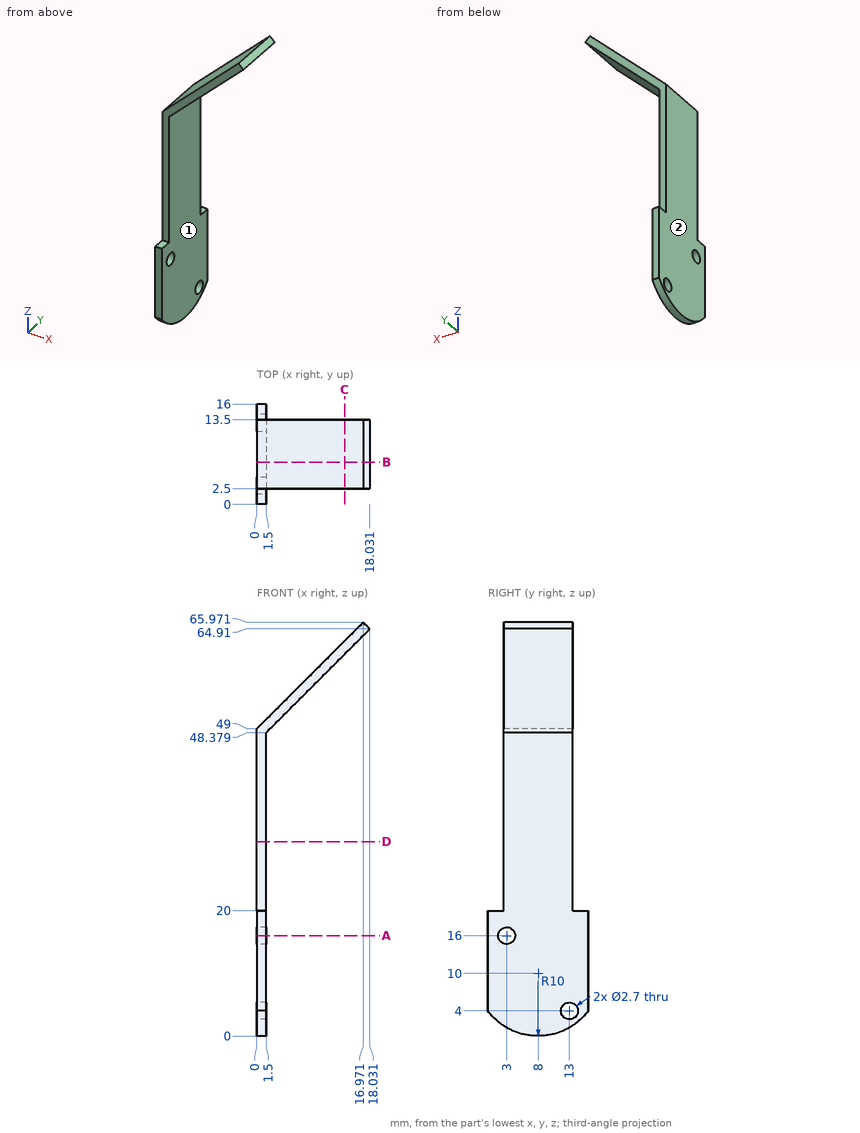
Part print with two shaded views. Sizes in mm from the minimum x, y, z corner. A direction names the side the tool comes from. Coordinates: 2 decimals unless noted, no trailing zeros. Write each loop counter-clockwise with the first axis right and the second up, starting at its lowest first coordinate (ties: lowest second). Pieces come first, ordered by that corner, then holes.
(1) Cut at A-A on z = 16. List the corners of the cut face in (x, y).
(2) Cut at B-B on y = 6.75. List the corners of the cut face in (x, z).
(3) Cut at C-C on x = 14. List the corners of the cut face in (y, z).
(4) Pin check, flat tips, straight feed: pin 1 Ø6 at (y, z) = (2, 21) entering from +X; pin 2 Ø9 at (x, z) = (12, 48.5) entering from -Y (3 decimals); pin 3 Ø5 at (y, z) = (7.5, 53.5) entering from +X; pin 4 Ø0.8 at (x, y) = (0.5, 15) entering from +Z. Stop position of each tip, or through.
(5) 3-axis set-ups, long thin cutter, end or side, ignore diameter. For the marked faces 1 and 2: which of +Z, -Z, +X, -X, +Y, -Y reach the whole face in a straight line?
(6) Drill centre lines: line 1 (X direction, y = 11, z = 46); line 2 (Z direction, x = 0.65, y = 3); line 3 (Z direction, x = 0.9, y = 3). Where is each one in solid material? Low to high.
(7) Cut at D-D on z = 31. List the corners of the cut face in (x, y).
Working result:
1. outline: (0, 0) - (1.5, 0) - (1.5, 1.65) - (0, 1.65) - close; (0, 4.35) - (1.5, 4.35) - (1.5, 16) - (0, 16) - close
2. outline: (0, 0.08) - (1.5, 0.08) - (1.5, 48.38) - (18.03, 64.91) - (16.97, 65.97) - (0, 49) - close
3. outline: (2.5, 60.88) - (13.5, 60.88) - (13.5, 63) - (2.5, 63) - close
4. pin 1: stops at x = 1.5
4. pin 2: passes through
4. pin 3: stops at x = 9.12
4. pin 4: stops at z = 20
5. face 1: -Z, +X, +Y, -Y
5. face 2: +Z, -Z, -X, +Y, -Y
6. line 1: x = 0 to 1.5
6. line 2: z = 1.34 to 14.65, 17.35 to 49.65
6. line 3: z = 1.34 to 14.65, 17.35 to 49.9
7. outline: (0, 2.5) - (1.5, 2.5) - (1.5, 13.5) - (0, 13.5) - close
